Read the model definition and answer for the solid it produces. Units are mm, in the model's axes. A direction names the side the tool comes from. Coordinates: 2 decimals unless noted, no trailing zeros. Loops run counter-clockwise (first coordinate to the right, second up) from the corner with the lowest first, then second, coordinate; pieces in that order, holes last.
from build123d import *

# Parameters (mm, degrees)
SKETCH1_W           = 22.352
SKETCH1_H           = 63.5
CUT_EXTRUDE2_START  = 11.176
SKETCH2_R           = 19.05
CUT_EXTRUDE2_DEPTH  = 102.671320188
CUT_EXTRUDE4_START  = 11.176
SKETCH3_R           = 4.3688
CUT_EXTRUDE4_DEPTH  = 127
CUT_EXTRUDE6_START  = 11.176
SKETCH4_R           = 6.7437
CUT_EXTRUDE6_DEPTH  = 9.652
CUT_EXTRUDE8_START  = 11.176
SKETCH5_R           = 4.3688
CUT_EXTRUDE8_DEPTH  = 127
CUT_EXTRUDE10_START = 11.176
SKETCH6_R           = 6.7437
CUT_EXTRUDE10_DEPTH = 9.652


with BuildPart() as part:
    # Sketch1 → Revolve1 (revolve)
    with BuildSketch(Plane(origin=(0, 0, 0), x_dir=(0, 1, 0), z_dir=(0, 0, 1)), mode=Mode.PRIVATE) as revolve1_sk:
        with Locations((0, 31.75)):
            Rectangle(SKETCH1_W, SKETCH1_H)
    revolve(revolve1_sk.sketch.rotate(Axis((0, -36.576, 0), (0, 1, 0)), 270), axis=Axis((0, -36.576, 0), (0, 1, 0)))

    # Sketch2 → Cut-Extrude2 (cut, through all)
    with BuildSketch(Plane(origin=(0, 0, 0), x_dir=(-1, 0, 0), z_dir=(0, 1, 0)).offset(CUT_EXTRUDE2_START)):
        with Locations(Location((0, 0, 0), (0, 0, 90))):
            Circle(SKETCH2_R)
    extrude(amount=-CUT_EXTRUDE2_DEPTH, mode=Mode.SUBTRACT)

    # Sketch3 → Cut-Extrude4 (cut)
    with BuildSketch(Plane(origin=(0, 0, 0), x_dir=(-1, 0, 0), z_dir=(0, 1, 0)).offset(CUT_EXTRUDE4_START)):
        with Locations(Location((53.975, 0, 0), (0, 0, 90))):
            Circle(SKETCH3_R)
    extrude(amount=-CUT_EXTRUDE4_DEPTH, mode=Mode.SUBTRACT)

    # Sketch4 → Cut-Extrude6 (cut)
    with BuildSketch(Plane(origin=(0, 0, 0), x_dir=(-1, 0, 0), z_dir=(0, 1, 0)).offset(CUT_EXTRUDE6_START)):
        with Locations(Location((53.975, 0, 0), (0, 0, 90))):
            Circle(SKETCH4_R)
    extrude(amount=-CUT_EXTRUDE6_DEPTH, mode=Mode.SUBTRACT)

    # Sketch5 → Cut-Extrude8 (cut)
    with BuildSketch(Plane(origin=(0, 0, 0), x_dir=(-1, 0, 0), z_dir=(0, 1, 0)).offset(CUT_EXTRUDE8_START)):
        with Locations(Location((0, 53.975, 0), (0, 0, 90))):
            Circle(SKETCH5_R)
        with Locations(Location((-53.975, 0, 0), (0, 0, 90))):
            Circle(SKETCH5_R)
        with Locations(Location((0, -53.975, 0), (0, 0, 90))):
            Circle(SKETCH5_R)
    extrude(amount=-CUT_EXTRUDE8_DEPTH, mode=Mode.SUBTRACT)

    # Sketch6 → Cut-Extrude10 (cut)
    with BuildSketch(Plane(origin=(0, 0, 0), x_dir=(-1, 0, 0), z_dir=(0, 1, 0)).offset(CUT_EXTRUDE10_START)):
        with Locations(Location((0, 53.975, 0), (0, 0, 90))):
            Circle(SKETCH6_R)
        with Locations(Location((-53.975, 0, 0), (0, 0, 90))):
            Circle(SKETCH6_R)
        with Locations(Location((0, -53.975, 0), (0, 0, 90))):
            Circle(SKETCH6_R)
    extrude(amount=-CUT_EXTRUDE10_DEPTH, mode=Mode.SUBTRACT)


solid = part.part
Item 1: Given pin 1 (8 mm diameter, centred on y = 5.5, z = -16, fed in from -X); pin 2 (7 mm diameter, centred on x = 0, z = -53.975, fed in from +Y); pin 3 (12 mm diameter, centred on y = 6, z = 4.5, fed in from +X); pin 4 (6.5 mm diameter, centred on x = 0.5, z = 56.5, fed in from +Y), each flat-ended and moving along its own axis, determine where each tip first touches the part or whether it passes through.
Numbers:
pin 1: stops at x = -62.36
pin 2: passes through
pin 3: stops at x = 63.5
pin 4: stops at y = 1.52
Item 2: Find the intervals of material crossed by line 1 along X through (y, z) = (6.5, 0); line 2 along X through (y, z) = (-6, 0); line 3 along X through (y, z) = (3.25, -48), in increasing order.
Numbers:
line 1: x = -63.5 to -60.72, -47.23 to -19.05, 19.05 to 47.23, 60.72 to 63.5
line 2: x = -63.5 to -58.34, -49.61 to -19.05, 19.05 to 49.61, 58.34 to 63.5
line 3: x = -41.57 to -3.13, 3.13 to 41.57
Item 3: A cutting plane is placed at D-D on z = 30. Determine the outline of the cut face in (x, y).
Numbers:
outline: (-55.97, -11.18) - (55.97, -11.18) - (55.97, 11.18) - (-55.97, 11.18) - close
Item 4: A cutting plane is placed at C-C on y = -9. Determine the outline of the cut face in (x, z) (3 decimals), then the cut area to 3 significant figures.
Numbers:
outline: circle Ø127 at (0, 0); hole circle Ø8.738 at (-53.975, 0); hole circle Ø38.1 at (0, 0); hole circle Ø8.738 at (0, -53.975); hole circle Ø8.738 at (0, 53.975); hole circle Ø8.738 at (53.975, 0)
area: 11,300 mm2
Item 5: Determine the mould class of faces 1 (the face through (61.99, 0.16, 13.77)), 2 (the face through (-49.643, -4.737, -0.569)), 3 (the face through (52.6, 1.524, 4.4)), 4 (the face through (-15, -11.176, 13)) for opening direction X: released by +X, released by -X, zero draft, split by the parting line, or undercut.
Numbers:
face 1: split by the parting line
face 2: undercut
face 3: undercut
face 4: zero draft
Item 6: A cutting plane is placed at B-B on z = 0. Determine the outline of the cut face in (x, y).
Numbers:
outline: (-63.5, -11.18) - (-58.34, -11.18) - (-58.34, 1.52) - (-60.72, 1.52) - (-60.72, 11.18) - (-63.5, 11.18) - close; (-49.61, -11.18) - (-19.05, -11.18) - (-19.05, 11.18) - (-47.23, 11.18) - (-47.23, 1.52) - (-49.61, 1.52) - close; (19.05, -11.18) - (49.61, -11.18) - (49.61, 1.52) - (47.23, 1.52) - (47.23, 11.18) - (19.05, 11.18) - close; (58.34, -11.18) - (63.5, -11.18) - (63.5, 11.18) - (60.72, 11.18) - (60.72, 1.52) - (58.34, 1.52) - close
Item 7: Which of the six approach directions +Z, -Z, +X, -X, +Y, -Y give full straight-line access (tool end or side, diameter ignored) to faces 5 (the face through (-4.4, 1.524, -52.6)), 6 (the face through (50.1, -4.74, 2.02))?
Numbers:
face 5: +Y
face 6: +Y, -Y
Item 8: A cutting plane is placed at A-A on x = 0. Determine the outline of the cut face in (y, z), then the cut area to 3 significant figures.
Numbers:
outline: (-11.18, -63.5) - (11.18, -63.5) - (11.18, -60.72) - (1.52, -60.72) - (1.52, -58.34) - (-11.18, -58.34) - close; (-11.18, -49.61) - (1.52, -49.61) - (1.52, -47.23) - (11.18, -47.23) - (11.18, -19.05) - (-11.18, -19.05) - close; (-11.18, 19.05) - (11.18, 19.05) - (11.18, 47.23) - (1.52, 47.23) - (1.52, 49.61) - (-11.18, 49.61) - close; (-11.18, 58.34) - (1.52, 58.34) - (1.52, 60.72) - (11.18, 60.72) - (11.18, 63.5) - (-11.18, 63.5) - close
area: 1,500 mm2
